Study the drawing (mm; zero at the part's minimum x, y, z) and answer. A direction names the side the tool comes from. Coordinates: 2 decimals unless noted, no trailing zeros. Order: outer loops, then holes, each group sorted by start corner. A loop starts at its lowest first (then second) coordinate and runs counter-clockwise, first axis right, second up. Notation, with made-up numbers: (76.5, -15) -> (106.5, -15) arc R26 cw to (106.5, 13) -> close; hole circle Ø6 at (-12, 69). An arc over 180 degrees is marked (long way). Answer in a Markdown table with one row per item. Add a question column.
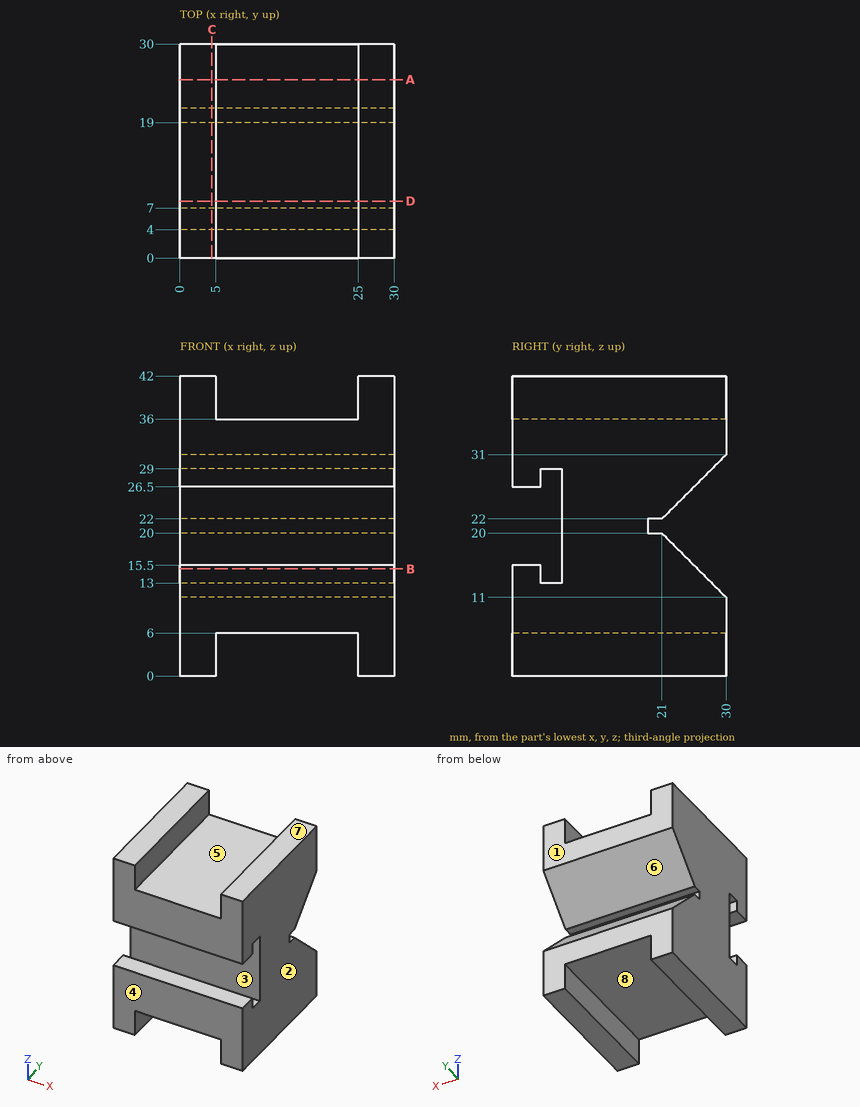
Q1. Given pin 1 (2 mm diameter, centred on x = 16.5, z = 27, fed in from +Y); pin 2 (8 mm diameter, centred on x = 13, y = 4.5, fed in from +Z); pin 3 (4.5 mm diameter, centred on x = 9, y = 1, fed in from -Z), each flat-ended and moving along its own axis, determine where each tip first touches the part or whether it passes through.
Q2. For the marked faces 5, 6, 7 and 8, determine the directions among +Z, -Z, +X, -X, +Y, -Y from which every point of the face is accessible in a straight line to the end or side of a thin tool.
Q3. Determine the mould class of the marked faces 1, 2, 3 and 4 for opening direction Y: +Y half, -Y half, draft (parallel to the pull), parting line (faces both ways), or undercut.
Q4. Straight lines are drawn through the part: line 1 (X direction, y = 15, z = 2.5); line 2 (Z direction, x = 12, y = 9.5); line 3 (Y direction, x = 19, z = 21). For each, find the intervals that lie inside material, in ascending order.
Q5. A cutting plane is placed at A-A (y = 25). Determine the outline of the cut face in (x, z).
Q6. A cutting plane is placed at C-C (x = 4.5). Determine the outline of the cut face in (y, z), then the cut area to 4 significant figures.
Q7. A cutting plane is placed at D-D (y = 8). Determine the outline of the cut face in (x, z).
Q8. A cutting plane is placed at B-B (z = 15). Determine the outline of the cut face in (x, y).
Returned:
| question | item | result |
|---|---|---|
| 1 | pin 1 | stops at y = 27 |
| 1 | pin 2 | stops at z = 36 |
| 1 | pin 3 | stops at z = 6 |
| 2 | face 5 | +Z, +Y, -Y |
| 2 | face 6 | +X, -X, +Y |
| 2 | face 7 | +Z, +X, -X, +Y, -Y |
| 2 | face 8 | -Z, +Y, -Y |
| 3 | face 1 | +Y half |
| 3 | face 2 | draft |
| 3 | face 3 | undercut |
| 3 | face 4 | -Y half |
| 4 | line 1 | x = 0 to 5, 25 to 30 |
| 4 | line 2 | z = 6 to 36 |
| 4 | line 3 | y = 7 to 19 |
| 5 | outline | (0, 0) -> (5, 0) -> (5, 6) -> (25, 6) -> (25, 0) -> (30, 0) -> (30, 16) -> (0, 16) -> close; (0, 26) -> (30, 26) -> (30, 42) -> (25, 42) -> (25, 36) -> (5, 36) -> (5, 42) -> (0, 42) -> close |
| 6 | outline | (0, 0) -> (30, 0) -> (30, 11) -> (21, 20) -> (19, 20) -> (19, 22) -> (21, 22) -> (30, 31) -> (30, 42) -> (0, 42) -> (0, 26.5) -> (4, 26.5) -> (4, 29) -> (7, 29) -> (7, 13) -> (4, 13) -> (4, 15.5) -> (0, 15.5) -> close |
| 6 | area | 1,065 mm² |
| 7 | outline | (0, 0) -> (5, 0) -> (5, 6) -> (25, 6) -> (25, 0) -> (30, 0) -> (30, 42) -> (25, 42) -> (25, 36) -> (5, 36) -> (5, 42) -> (0, 42) -> close |
| 8 | outline | (0, 0) -> (30, 0) -> (30, 4) -> (0, 4) -> close; (0, 7) -> (30, 7) -> (30, 26) -> (0, 26) -> close |
